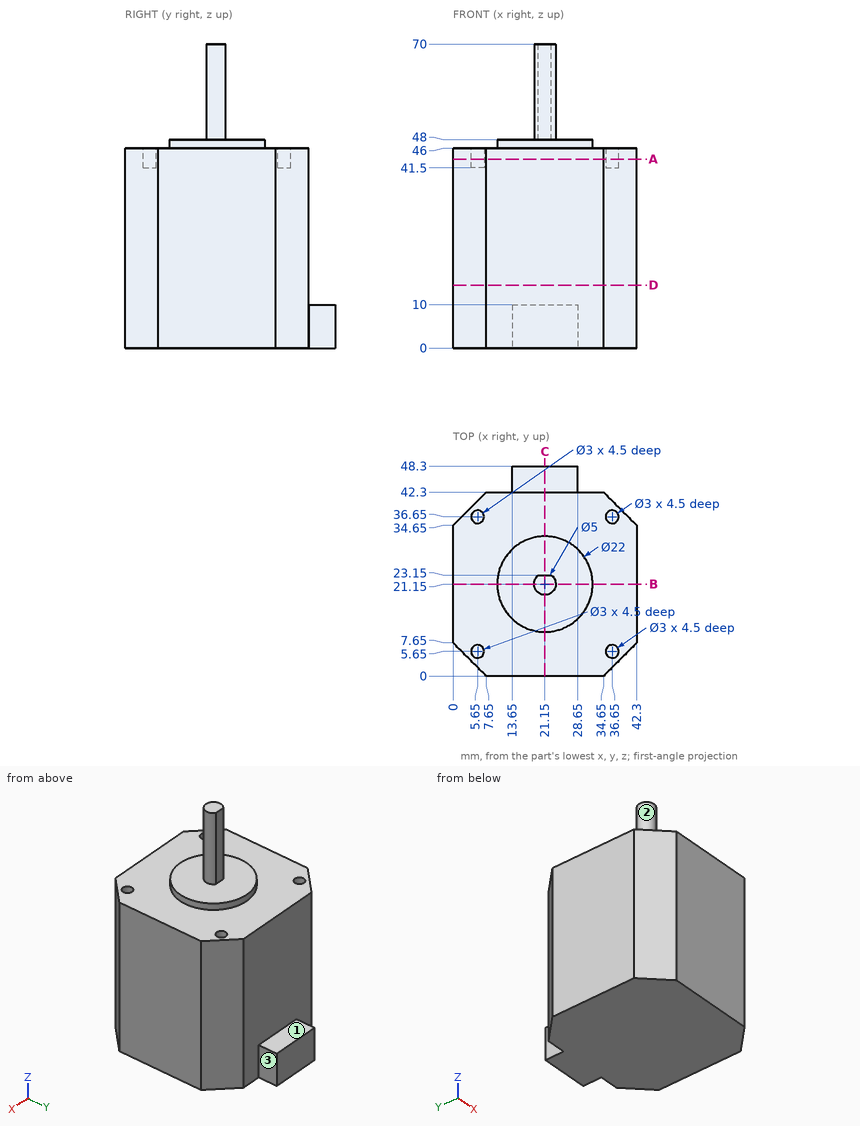
Study the drawing (mm; zero at the part's minimum x, y, z) and answer. A direction names the side the tool comes from. Round coordinates to 2 decimals unless told otherwise and drop trailing zeros. Loops run counter-clockwise (first coordinate to the right, second up) from the corner with the lowest first, then second, coordinate; pieces in that order, holes last. Notation, with made-up numbers: (-34, 73.5) -> (21, 73.5) arc R32 cw to (21, 104.5) -> close; hole circle Ø2 at (-29, 18.5). An arc over 180 degrees is marked (long way). Use one line per item in the form item = value.
1. Flat-ended cylindrical pins translate along their axes: pin 1 Ø3.5 at (x, y) = (5, 36) entering from +Z; pin 2 Ø12 at (y, z) = (15.5, 53.5) entering from +X; pin 3 Ø3 at (x, y) = (18.5, 45.5) entering from +Z. Find the tip coordinate at first contact, or state that the pin passes through.
Answer key:
pin_1 = 46
pin_2 = 31.66
pin_3 = 10
2. The part is cut by section D-D on z = 14.5. Determine the outline of the cut face in (x, y), and give its area (3 significant figures).
Answer key:
outline = (0, 7.65) -> (7.65, 0) -> (34.65, 0) -> (42.3, 7.65) -> (42.3, 34.65) -> (34.65, 42.3) -> (7.65, 42.3) -> (0, 34.65) -> close
area = 1,670 mm²
3. The part is cut by section C-C on x = 21.15. Determine the outline of the cut face in (y, z), and give its area (3 significant figures).
Answer key:
outline = (0, 0) -> (48.3, 0) -> (48.3, 10) -> (42.3, 10) -> (42.3, 46) -> (32.15, 46) -> (32.15, 48) -> (23.15, 48) -> (23.15, 70) -> (18.65, 70) -> (18.65, 48) -> (10.15, 48) -> (10.15, 46) -> (0, 46) -> close
area = 2,150 mm²
4. Find the intervals of material crossed by probe 1 along X at (y, z) = (36, 44); probe 2 along Y at (x, z) = (5, 43); probe 3 along Z at (x, y) = (17.5, 38), in increasing order. Write a range as [from, to].
Answer key:
probe_1 = [1.35, 4.3], [7, 35.3], [38, 40.95]
probe_2 = [2.65, 4.3], [7, 35.3], [38, 39.65]
probe_3 = [0, 46]
5. A tool of negligible diameter and unlimited length cuts with its end or side. For the marked faces 1, 2 and 3, from which of +Z, -Z, +X, -X, +Y, -Y can it reach the whole face along a straight path? Write none if from no direction.
Answer key:
face_1 = +Z, +X, -X, +Y
face_2 = +Z
face_3 = +Z, -Z, +X, +Y
6. The part is cut by section A-A on z = 43.5. Determine the outline of the cut face in (x, y).
Answer key:
outline = (0, 7.65) -> (7.65, 0) -> (34.65, 0) -> (42.3, 7.65) -> (42.3, 34.65) -> (34.65, 42.3) -> (7.65, 42.3) -> (0, 34.65) -> close; hole circle Ø3 at (5.65, 5.65); hole circle Ø3 at (5.65, 36.65); hole circle Ø3 at (36.65, 5.65); hole circle Ø3 at (36.65, 36.65)
7. The part is cut by section B-B on y = 21.15. Determine the outline of the cut face in (x, z), and give its area (3 significant figures).
Answer key:
outline = (0, 0) -> (42.3, 0) -> (42.3, 46) -> (32.15, 46) -> (32.15, 48) -> (23.65, 48) -> (23.65, 70) -> (18.65, 70) -> (18.65, 48) -> (10.15, 48) -> (10.15, 46) -> (0, 46) -> close
area = 2,100 mm²
